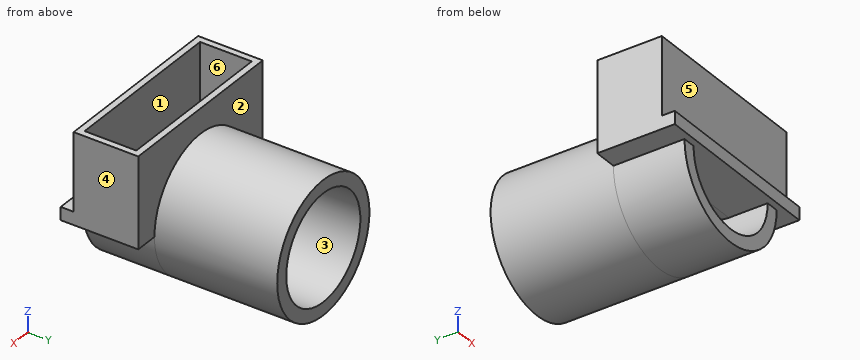
```python
from build123d import *
from build123d.topology import SkipClean

# Parameters (mm, degrees)
SKETCH_2_R          = 259.207
SKETCH_2_R_2        = 208.407
F_19MM_DEPTH        = 482.6
F_11MM_START        = -279.4
F_11MM_DEPTH        = 279.4
SKETCH_8_W          = 700.278
SKETCH_8_H          = 254
EXTRUDE_2_DEPTH     = 355.6
SKETCH_11_W         = 649.478
SKETCH_11_H         = 203.2
CUT_EXTRUDE_1_DEPTH = 279.4
FILLET_2_R          = 127
SKETCH_13_W         = 700.278
SKETCH_13_H         = 50.8
F_2MM_DEPTH         = 50.8


with BuildPart() as part:
    # 草圖2 → 主件固定 19mm (new body)
    with BuildSketch(Plane(origin=(0, 0, 0), x_dir=(1, 0, 0), z_dir=(0, 1, 0))):
        Circle(SKETCH_2_R)
        Circle(SKETCH_2_R_2, mode=Mode.SUBTRACT)
    extrude(amount=F_19MM_DEPTH)

    # 草圖3 → 下填充 11mm (add)
    with SkipClean():  # the faces are left unmerged after this step: merging them gives an invalid solid
        with BuildSketch(Plane(origin=(0, 0, 0), x_dir=(1, 0, 0), z_dir=(0, 1, 0)).offset(F_11MM_START)):
            with BuildLine():
                ThreePointArc((208.407, 0), (0, 208.407), (-208.407, 0))
                Line((-208.407, 0), (-259.207, 0))
                ThreePointArc((-259.207, 0), (0, 259.207), (259.207, 0))
                Line((259.207, 0), (208.407, 0))
            make_face()
        extrude(amount=F_11MM_DEPTH)

    # 草圖8 → 填料-伸長2 (add)
    with SkipClean():  # the faces are left unmerged after this step: merging them gives an invalid solid
        with BuildSketch(Plane.XY):
            with Locations((0, -127)):
                Rectangle(SKETCH_8_W, SKETCH_8_H)
        extrude(amount=EXTRUDE_2_DEPTH)

    # 草圖11 → 除料-伸長1 (cut)
    with SkipClean():  # the faces are left unmerged after this step: merging them gives an invalid solid
        with BuildSketch(Plane.XY.offset(355.6)):
            with Locations((0, -127)):
                Rectangle(SKETCH_11_W, SKETCH_11_H)
        extrude(amount=-CUT_EXTRUDE_1_DEPTH, mode=Mode.SUBTRACT)

    # 圓角2
    # the kernel refuses this fillet: 127 mm, written as the material it takes off along each edge
    with BuildSketch(Plane(origin=(-525.907, 0, 0), x_dir=(0, 0, 1), z_dir=(1, 0, 0))) as fillet_2_piece_1_section:
        with BuildLine():
            CenterArc((FILLET_2_R, FILLET_2_R), FILLET_2_R, 180, 90)
            Line((0, FILLET_2_R), (0, 0))
            Line((0, 0), (FILLET_2_R, 0))
        make_face()
    fillet_2_piece_1 = extrude(amount=1051.814, mode=Mode.PRIVATE)
    fillet_2_piece_1 = fillet_2_piece_1 & Plane(origin=(0, -28.656065258, 0), x_dir=(1, 0, 0), z_dir=(0, -1, 0)) * Cylinder(208.407, 2612, mode=Mode.PRIVATE)
    add(fillet_2_piece_1, mode=Mode.SUBTRACT)

    # 草圖13 → 防水凸出2mm (add)
    with BuildSketch(Plane.XZ.offset(254)):
        with Locations((0, 25.4)):
            Rectangle(SKETCH_13_W, SKETCH_13_H)
    extrude(amount=F_2MM_DEPTH)


solid = part.part
```
Verification items for the finished model (mm, model axes). Face numbers are marked on the shaded views. A direction names the side the tool comes from. Give positions to 0.01 mm unless a question says otherwise; leave off trailing zeros. Order: outer loops, then holes, each group sorted by start corner. A loop starts at its lowest first (then second) coordinate and runs counter-clockwise, first axis right, second up. Notation, with made-up numbers: M -38,-25 L 1,-25 A23 cw 1,-5 Z; hole C 18.25,-16 d4. An arc over 180 degrees is marked long. Return JSON: item names as keys, results as strings. Group by question number.
1) Section check A-A on x = 0. Record the cut outline in (y, z).
2) Scan lines: line 1 (X direction, y = 101, z = 0); line 2 (Y direction, x = 8.5, z = 329.5). Record each from-to range of solid material in increasing order.
3) Section check B-B on z = -103. Record the cut outline in (x, y), and give its area (3 significant figures).
4) Go/stop test with flat-tipped pins: pin 1 Ø10 at (x, y) = (76.5, 123.5) entering from -Z; pin 2 Ø4 at (x, y) = (154.5, -222) entering from -Z; pin 3 Ø3 at (x, z) = (-163, 55) entering from -Y. Record where each tip stops, or that it passes through.
5) Mould release check, pull along X, two halves, no side actions. Record for the marked faces 4, 5 and 6: pulls with the +X half, pulls with the -X half, needs draft (parallel to the pull), parting line crosses it, or undercut.
6) Section check D-D on z = 166. Record the cut outline in (x, y), and give its area (3 significant figures).
7) Access from +Z, -Z, +X, -X, +Y, -Y to the whole of each face (thin tool, end or side, straight path). Record for the marked faces 1, 2 and 3.
Answer block:
{
 "1": {"outline": "M -304.8,0 L -127,0 A127 ccw 0,127 L 0,208.41 L 482.6,208.41 L 482.6,259.21 L 0,259.21 L 0,355.6 L -25.4,355.6 L -25.4,76.2 L -228.6,76.2 L -228.6,355.6 L -254,355.6 L -254,50.8 L -304.8,50.8 Z; M -279.4,-259.21 L 482.6,-259.21 L 482.6,-208.41 L -279.4,-208.41 Z"},
 "2": {"line 1": "x = -259.21 to -208.41, 208.41 to 259.21", "line 2": "y = -254 to -228.6, -25.4 to 0"},
 "3": {"outline": "M -237.86,-279.4 L -181.18,-279.4 L -181.18,482.6 L -237.86,482.6 Z; M 181.18,-279.4 L 237.86,-279.4 L 237.86,482.6 L 181.18,482.6 Z", "area": "86,400 mm^2"},
 "4": {"pin 1": "stops at z = -249.15", "pin 2": "stops at z = -209.6", "pin 3": "stops at y = -254"},
 "5": {"face 4": "pulls with the +X half", "face 5": "needs draft", "face 6": "undercut"},
 "6": {"outline": "M -350.14,-254 L 350.14,-254 L 350.14,0 L 199.08,0 L 199.08,482.6 L 126.01,482.6 L 126.01,0 L -126.01,0 L -126.01,482.6 L -199.08,482.6 L -199.08,0 L -350.14,0 Z; hole M -324.74,-228.6 L 324.74,-228.6 L 324.74,-25.4 L -324.74,-25.4 Z", "area": "116,000 mm^2"},
 "7": {"face 1": "+Z", "face 2": "+Z, +Y", "face 3": "+Y"}
}
